Verification items for this drawing (mm, ordinates from the low corner). Round coordinates to 2 decimals unless told otherwise and drop trailing zeros. Loops run counter-clockwise (first coordinate to the right, second up) from the corner with the lowest first, then second, coordinate; pieces in that order, holes last. Notation, with made-up numbers: (-36, 59) -> (-13, 59) arc R22 cw to (-13, 72) -> close; hole circle Ø7 at (88, 2.25). An arc over 180 degrees is marked (long way). Use a Markdown table: item, result. Add a question column.
Q1. Gauge pin test, flat ends, axial feed: P1, Ø1.5, axis at x = 15.5, z = 5, coming from the -Y side; P2, Ø3.5, axis at x = 7, z = 4, coming from the +Y side; P3, Ø1, axis at y = 18.5, z = 1, coming from the +X side; P4, Ø4, axis at x = 37, z = 4, coming from the -Y side. Record the tip position at first contact, or that the pin passes through.
Q2. Sectioned sample at B-B, the plane x = 7. Enter the section's corners in (y, z), then the cut area to 3 significant figures.
Q3. Sectioned sample at C-C, the plane z = 7. Enter the section's corners in (x, y), then the cut area to 3 significant figures.
Q4. Sectioned sample at A-A, the plane z = 4. Enter the section's corners in (x, y).
Q5. Material ranges on L1, parallel to X at y = 38.75, z = 4; L2, parallel to Z at x = 37, y = 6; L3, parallel to Z at x = 8.5, y = 8, recorded low to high.
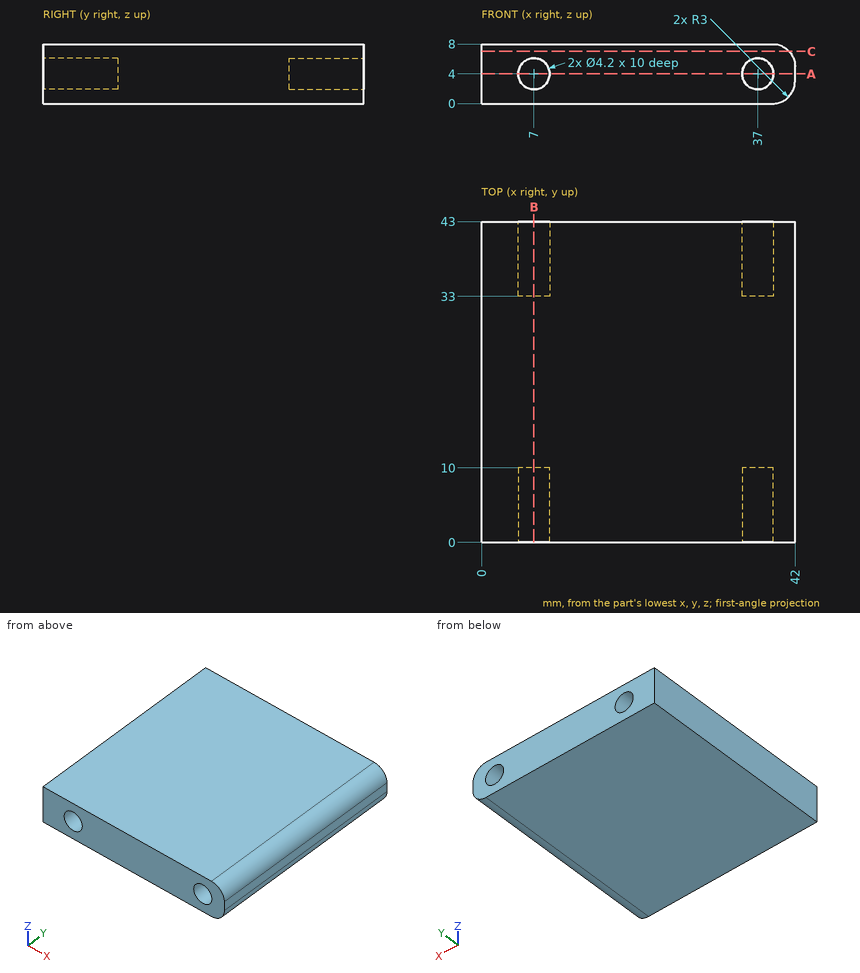
Values:
| question | item | result |
|---|---|---|
| 1 | P1 | y = 0 |
| 1 | P2 | y = 33 |
| 1 | P3 | x = 41.6 |
| 1 | P4 | y = 10 |
| 2 | outline | (0, 0) -> (43, 0) -> (43, 1.9) -> (33, 1.9) -> (33, 6.1) -> (43, 6.1) -> (43, 8) -> (0, 8) -> (0, 6.1) -> (10, 6.1) -> (10, 1.9) -> (0, 1.9) -> close |
| 2 | area | 260 mm^2 |
| 3 | outline | (0, 0) -> (41.24, 0) -> (41.24, 43) -> (0, 43) -> close |
| 3 | area | 1,770 mm^2 |
| 4 | outline | (0, 0) -> (4.9, 0) -> (4.9, 10) -> (9.1, 10) -> (9.1, 0) -> (34.9, 0) -> (34.9, 10) -> (39.1, 10) -> (39.1, 0) -> (42, 0) -> (42, 43) -> (39.1, 43) -> (39.1, 33) -> (34.9, 33) -> (34.9, 43) -> (9.1, 43) -> (9.1, 33) -> (4.9, 33) -> (4.9, 43) -> (0, 43) -> close |
| 5 | L1 | 0 to 4.9, 9.1 to 34.9, 39.1 to 42 |
| 5 | L2 | 0 to 1.9, 6.1 to 8 |
| 5 | L3 | 0 to 2.53, 5.47 to 8 |
